Check sheet for the drawn part. Datum: minimum x, y, z corner. Units: mm. A direction names the side the tool comes from. Round coordinates to 2 decimals unless told otherwise and drop trailing zeros. Order: outer loops, then holes, each group sorted by start corner. A loop starts at its lowest first (then second) coordinate and runs counter-clockwise, first axis right, second up. Notation, with made-up numbers: M 10.5,75 L 27.5,75 A14 ccw 27.5,84 Z; hole C 38,-10.5 d8. An arc over 180 degrees is marked long. Answer as a JSON object with one key per item and string values. Group by question number.
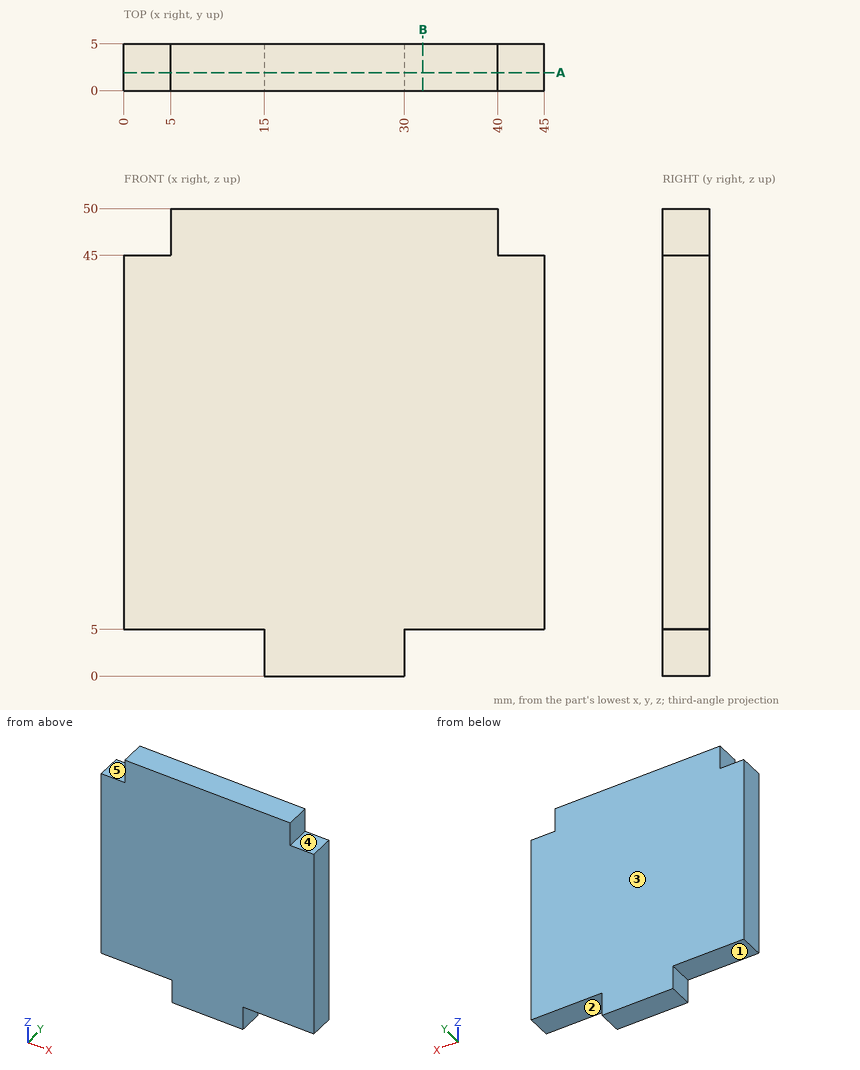
1) Go/stop test with flat-tipped pins: P1, Ø2.5, axis at x = 7, y = 3.5, coming from the -Z side; P2, Ø2.5, axis at y = 1.5, z = 46.5, coming from the -X side; P3, Ø1.5, axis at x = 42, y = 1.5, coming from the +Z side. Record where each tip stops, or that it passes through.
2) Set-up check for the marked faces 1, 2, 3, 4 and 5: record each of +Z, -Z, +X, -X, +Y, -Y from which the full face is reachable in a straight line by a thin tool's end or side.
3) Sectioned sample at B-B (x = 32). Record the boundary of the cut face in (y, z), then the cut area to 3 significant figures.
4) Sectioned sample at A-A (y = 1.95). Record the boundary of the cut face in (x, z).
5) Thickness scan on line 1 along Z through (x, y) = (41, 3.7); line 2 along Z through (x, y) = (7, 2.4); line 3 along X through (y, z) = (1.45, 48.5). Record the ranges inside material, lowest first. Write a range as [from, to].
Final values:
{
 "1": {"P1": "stops at z = 5", "P2": "stops at x = 5", "P3": "stops at z = 45"},
 "2": {"face 1": "-Z, -X, +Y, -Y", "face 2": "-Z, +X, +Y, -Y", "face 3": "+Z, -Z, +X, -X, +Y", "face 4": "+Z, +X, +Y, -Y", "face 5": "+Z, -X, +Y, -Y"},
 "3": {"outline": "M 0,5 L 5,5 L 5,50 L 0,50 Z", "area": "225 mm^2"},
 "4": {"outline": "M 0,5 L 15,5 L 15,0 L 30,0 L 30,5 L 45,5 L 45,45 L 40,45 L 40,50 L 5,50 L 5,45 L 0,45 Z"},
 "5": {"line 1": "z = [5, 45]", "line 2": "z = [5, 50]", "line 3": "x = [5, 40]"}
}
